from build123d import *

# Parameters (mm, degrees)
SKETCH1_R             = 25
SKETCH1_R_2           = 12.7
SKETCH1_R_3           = 6.35
BOSS_EXTRUDE1_DEPTH   = 5.6
F_5_0MM_DOWEL_HOLE2_D = 5
F_5_0MM_DOWEL_HOLE3_D = 5
SKETCH10_R            = 12.7
CUT_EXTRUDE1_DEPTH    = 20


with BuildPart() as part:
    # Sketch1 → Boss-Extrude1 (new body)
    with BuildSketch(Plane.XZ):
        with BuildLine():
            ThreePointArc((-51.817317458, -193.490941341), (0, -235.814796706), (51.817317458, -193.490941341))
            ThreePointArc((51.817317458, -193.490941341), (56.278810161, -184.410921807), (64.613246931, -178.676042941))
            ThreePointArc((64.613246931, -178.676042941), (0, 190), (-64.613246931, -178.676042941))
            ThreePointArc((-64.613246931, -178.676042941), (-56.278810161, -184.410921807), (-51.817317458, -193.490941341))
        make_face()
        Circle(SKETCH1_R, mode=Mode.SUBTRACT)
        with Locations((0, 100)):
            Circle(SKETCH1_R_2, mode=Mode.SUBTRACT)
        with Locations((-0.009704669, -179.999999411)):
            Circle(SKETCH1_R_3, mode=Mode.SUBTRACT)
    extrude(amount=BOSS_EXTRUDE1_DEPTH)

    # Ø5.0mm Dowel Hole2 (through all)
    with Locations(Plane(origin=(0, 0, 0), x_dir=(1, 0, 0), z_dir=(0, 1, 0))):
        with Locations((-147.224318643, 85)):
            Hole(F_5_0MM_DOWEL_HOLE2_D / 2)

    # Ø5.0mm Dowel Hole3 (through all)
    with Locations(Plane(origin=(0, 0, 0), x_dir=(1, 0, 0), z_dir=(0, 1, 0))):
        with Locations((-170, 0), (-140, 0), (-147.224318643, 85), (-70, 121.24355653), (-85, 147.224318643), (85, 147.224318643), (70, 121.24355653), (147.224318643, 85), (140, 0), (170, 0), (147.224318643, -85), (70, -121.24355653), (85, -147.224318643), (-85, -147.224318643), (-70, -121.24355653), (-20, -34.641016151), (20, -34.641016151), (40, 0), (-40, 0), (-20, 34.641016151), (20, 34.641016151), (-147.224318643, -85), (0, -170)):
            Hole(F_5_0MM_DOWEL_HOLE3_D / 2)

    # Sketch10 → Cut-Extrude1 (cut)
    with BuildSketch(Plane(origin=(0, 0, 0), x_dir=(-1, 0, 0), z_dir=(0, 1, 0))):
        with Locations((0, 100)):
            Circle(SKETCH10_R)
        with Locations((86.602540378, 50)):
            Circle(SKETCH10_R)
        with Locations((86.602540378, -50)):
            Circle(SKETCH10_R)
        with Locations((0, -100)):
            Circle(SKETCH10_R)
        with Locations((-86.602540378, -50)):
            Circle(SKETCH10_R)
        with Locations((-86.602540378, 50)):
            Circle(SKETCH10_R)
    extrude(amount=-CUT_EXTRUDE1_DEPTH, mode=Mode.SUBTRACT)


solid = part.part
Work out the finished part from the listing and answer in its coordinate system (mm). Coordinates: 2 decimals unless noted, no trailing zeros. Write each loop counter-clockwise with the first axis right and the second up, starting at its lowest first coordinate (ties: lowest second). Pieces come first, ordered by that corner, then holes. Notation, with made-up numbers: M 55,64 L 77,64 A8 ccw 77,77 Z; hole C 88.5,19 d11. An arc over 180 degrees is marked long. Write item = value, one per line.
1. The part is cut by section D-D (z = 57). Determine the outline of the cut face in (x, y).
Solution:
outline = M -181.25,-5.6 L -97.2,-5.6 L -97.2,0 L -181.25,0 Z; M -76.01,-5.6 L 76.01,-5.6 L 76.01,0 L -76.01,0 Z; M 97.2,-5.6 L 181.25,-5.6 L 181.25,0 L 97.2,0 Z
2. The part is cut by section A-A (z = -100). Determine the outline of the cut face in (x, y), then the cut area to 3 significant figures.
Solution:
outline = M -161.55,-5.6 L -12.7,-5.6 L -12.7,0 L -161.55,0 Z; M 12.7,-5.6 L 161.55,-5.6 L 161.55,0 L 12.7,0 Z
area = 1,670 mm2
3. Straight lines are drawn through the part: line 1 (X direction, y = -1.75, z = 85); line 2 (Z direction, x = -82, y = -4.2); line 3 (X direction, y = -2.2, z = -145). For each, find the intervals that lie inside material, in ascending order. Write a range as from..to.
Solution:
line_1 = -169.93..-149.72, -144.72..144.72, 149.72..169.93
line_2 = -171.39..-61.84, -38.16..38.16, 61.84..171.39
line_3 = -122.78..-86.14, -83.86..83.86, 86.14..122.78
4. Flat-ended cylindrical pins translate along their axes: pin 1 (20.5 mm diameter, centred on x = 86.6, z = 50, fed in from +Y); pin 2 (1 mm diameter, centred on x = 39, y = -3, fed in from -Z); pin 3 (2 mm diameter, centred on x = 15, y = -4.5, fed in from +Z); pin 4 (1.5 mm diameter, centred on x = -92.5, y = -4, fed in from -Z). Find the tip coordinate at first contact, or state that the pin passes through.
Solution:
pin_1 = through
pin_2 = -219.19
pin_3 = 189.48
pin_4 = -166.38
5. The part is cut by section C-C (y = -3.5). State how many separate pieces and enclosed holes the cut face has, then the cut area to 3 significant figures.
Solution:
separate_pieces = 1
enclosed_holes = 31
area = 112,000 mm2
6. The part is cut by section B-B (z = -50). Determine the outline of the cut face in (x, y), then the cut area to 3 significant figures.
Solution:
outline = M -183.3,-5.6 L -99.3,-5.6 L -99.3,0 L -183.3,0 Z; M -73.9,-5.6 L 73.9,-5.6 L 73.9,0 L -73.9,0 Z; M 99.3,-5.6 L 183.3,-5.6 L 183.3,0 L 99.3,0 Z
area = 1,770 mm2
